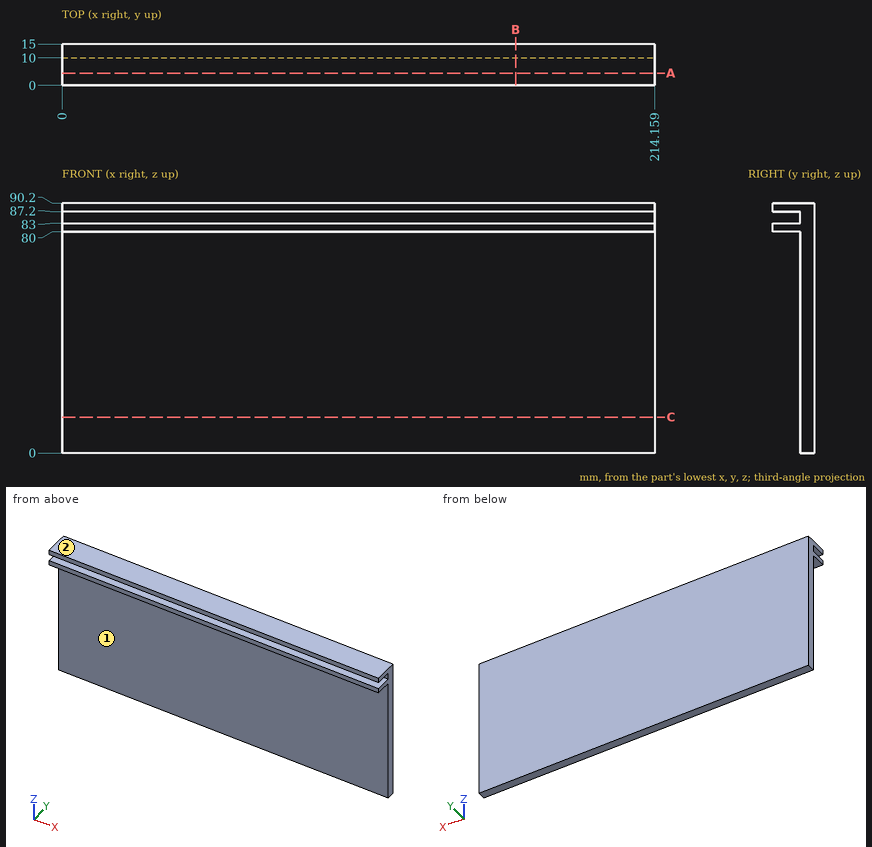
Source: three-view drawing plus pictorial views. Frame: mm from the lowest corner of the part. A direction names the side the tool comes from. Give positions to 0.01 mm unless a question says otherwise; leave off trailing zeros. Loops run counter-clockwise (first coordinate to the right, second up) from the corner with the lowest first, then second, coordinate; pieces in that order, holes last. Notation, with made-up numbers: (49.25, 18.25) -> (79.25, 18.25) arc R22 ccw to (79.25, 30.25) -> close; hole circle Ø10 at (-2, -5). An arc over 180 degrees is marked (long way). Put each result on its own line as item: value. Start each with the question number.
1) Cut plane A-A (y = 4.5). Return loops of the section in (x, z).
2) Reachability of the marked faces 1 and 2 from +Z, -Z, +X, -X, +Y, -Y: full face, straight path, thin tool, end or side. Return the list, or none.
3) Cut plane C-C (z = 13). Return loops of the section in (x, y).
4) Cut plane B-B (x = 164). Return loops of the section in (y, z).
5) Material intervals for probe 1 along Z at (x, y) = (105, 8.5); probe 2 along Y at (x, z) = (83, 59), sorted ascending.
6) Contact query for flat-ended pins moving along their axis: P1, Ø10, axis at x = 127.5, z = 19, coming from the -Y side; P2, Ø3, axis at x = 189, y = 2, coming from the -Z side. Output: stop coordinate, or through.
Results are:
1. outline: (0, 80) -> (214.16, 80) -> (214.16, 83) -> (0, 83) -> close; (0, 87.2) -> (214.16, 87.2) -> (214.16, 90.2) -> (0, 90.2) -> close
2. face 1: -Z, +X, -X, -Y
2. face 2: +Z, +X, -X, +Y, -Y
3. outline: (0, 10) -> (214.16, 10) -> (214.16, 15) -> (0, 15) -> close
4. outline: (0, 80) -> (10, 80) -> (10, 0) -> (15, 0) -> (15, 90.2) -> (0, 90.2) -> (0, 87.2) -> (10, 87.2) -> (10, 83) -> (0, 83) -> close
5. probe 1: z = 80 to 83, 87.2 to 90.2
5. probe 2: y = 10 to 15
6. P1: stops at y = 10
6. P2: stops at z = 80
